Design review of the part shown in the three views and the two pictorial views. Dimensions are in mm from the part's minimum x, y and z. Coordinates: 2 decimals unless noted, no trailing zeros. Loops run counter-clockwise (first coordinate to the right, second up) from the corner with the lowest first, then second, coordinate; pieces in that order, holes last. Notation, with made-up numbers: M -21,77 L -6,77 A14 ccw -6,88 Z; hole C 37,-6.5 d1. An arc over 180 degrees is marked long. Answer as a JSON object with one key per item and string values. Group by question number.
Item 1: Wall thickness on L1, parallel to X at y = 2.5, z = 59 (1 decimal); L2, parallel to Y at x = 3.2, z = 58.5; L3, parallel to Y at x = 0.6, z = 58.5 (1 decimal): over which ranges is each line inside the solid? List them lowest first. Write a range as from..to.
Item 2: Add section C-C (y = 0.7). State the section outline as (x, z) points (1 decimal), then the cut area to 3 significant figures.
Item 3: Add section A-A (z = 25.5). State the section outline as (x, y) points.
Item 4: Add section B-B (x = 0.65). State the section outline as (y, z) points (1 decimal), then the cut area to 3 significant figures.
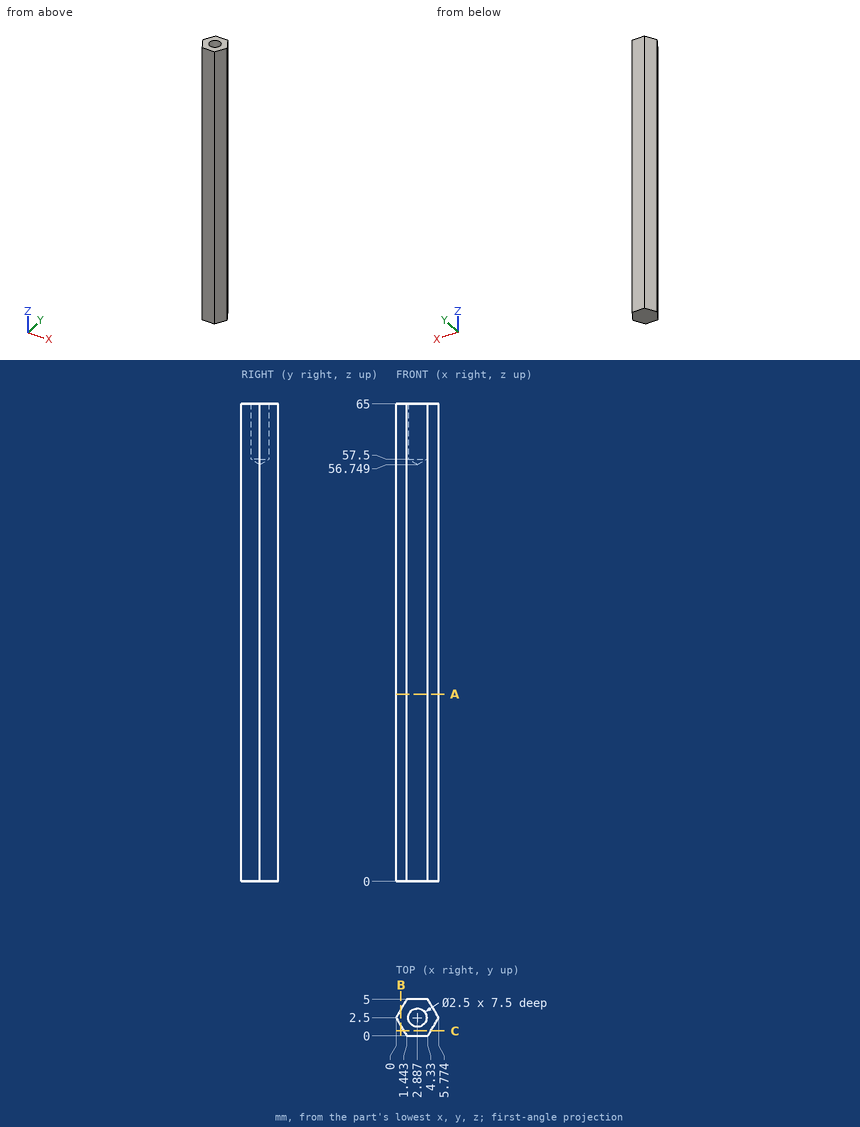
From the geometry:
{
 "1": {"L1": "x = 0..1.6, 4.1..5.8", "L2": "y = 0..1.29, 3.71..5", "L3": "y = 1.5..3.5"},
 "2": {"outline": "M 1,0 L 4.7,0 L 4.7,65 L 1,65 Z", "area": "240 mm²"},
 "3": {"outline": "M 0,2.5 L 1.44,0 L 4.33,0 L 5.77,2.5 L 4.33,5 L 1.44,5 Z"},
 "4": {"outline": "M 1.4,0 L 3.6,0 L 3.6,65 L 1.4,65 Z", "area": "146 mm²"}
}
